from build123d import *

# Parameters (mm, degrees)
SKETCH_1_W          = 30
SKETCH_1_H          = 22
EXTRUDE_1_DEPTH     = 1
SKETCH_2_R          = 0.5
SKETCH_2_R_2        = 0.75
CUT_EXTRUDE_1_DEPTH = 38.215588132
SKETCH_3_W          = 3
SKETCH_3_H          = 10
EXTRUDE_2_DEPTH     = 1
SKETCH_4_R          = 0.5
CUT_EXTRUDE_2_DEPTH = 1


with BuildPart() as part:
    # ｽｹｯﾁ1 → ﾎﾞｽ - 押し出し1 (new body)
    with BuildSketch(Plane.XY):
        with Locations((15, 11)):
            Rectangle(SKETCH_1_W, SKETCH_1_H)
    extrude(amount=EXTRUDE_1_DEPTH)

    # ｽｹｯﾁ2 → ｶｯﾄ - 押し出し1 (cut, through all)
    with BuildSketch(Plane.XY.offset(1)):
        with Locations((4, 17.25)):
            Circle(SKETCH_2_R)
        with Locations((4, 14.71)):
            Circle(SKETCH_2_R)
        with Locations((4, 12.17)):
            Circle(SKETCH_2_R)
        with Locations((4, 9.63)):
            Circle(SKETCH_2_R)
        with Locations((4, 7.09)):
            Circle(SKETCH_2_R)
        with Locations((4, 4.55)):
            Circle(SKETCH_2_R)
        with Locations((26.19, 18.69)):
            Circle(SKETCH_2_R_2)
        with Locations((26.19, 13.61)):
            Circle(SKETCH_2_R_2)
        with Locations((26.19, 8.53)):
            Circle(SKETCH_2_R_2)
        with Locations((26.19, 3.45)):
            Circle(SKETCH_2_R_2)
    extrude(amount=-CUT_EXTRUDE_1_DEPTH, mode=Mode.SUBTRACT)

    # ｽｹｯﾁ3 → ﾎﾞｽ - 押し出し2 (add)
    with BuildSketch(Plane.XY.offset(1)):
        with Locations((15.5, 11)):
            Rectangle(SKETCH_3_W, SKETCH_3_H)
    extrude(amount=EXTRUDE_2_DEPTH)

    # ｽｹｯﾁ4 → ｶｯﾄ - 押し出し2 (cut)
    with BuildSketch(Plane.XY.offset(2)):
        with Locations((15.5, 6)):
            Circle(SKETCH_4_R)
    extrude(amount=-CUT_EXTRUDE_2_DEPTH, mode=Mode.SUBTRACT)


solid = part.part
Design review of the part built by this model. Coordinates are the model's own, in mm. A direction names the side the tool comes from. Coordinates: 2 decimals unless noted, no trailing zeros. Loops run counter-clockwise (first coordinate to the right, second up) from the corner with the lowest first, then second, coordinate; pieces in that order, holes last. Notation, with made-up numbers: M 16.25,-35 L 45.25,-35 A25 ccw 45.25,-14 Z; hole C -6,-3 d5. An arc over 180 degrees is marked long. Use one line per item in the form item = value.
(1) Clearance check with flat-ended pins moving along their axes: P1, Ø0.5, axis at y = 11, z = 1.5, coming from the -X side; P2, Ø1.1, axis at y = 12.5, z = 1.5, coming from the +X side; P3, Ø0.5, axis at x = 16.5, z = 1.5, coming from the -Y side; P4, Ø6.5, axis at x = 21.5, y = 15, coming from the +Z side. State where each tip first meets the part, or that it passes through.
Return value:
P1 = 14
P2 = 30
P3 = 6
P4 = 1
(2) For faces 1 (the face through (17, 10.9, 1.5)), 2 (the face through (15.5, 16, 1.5)), 3 (the face through (15.5, 6.5, 1.5)), 4 (the face through (14, 10.9, 1.5)), list the 3-axis set-ups (+Z, -Z, +X, -X, +Y, -Y) from which the entire face can be reached by the end or side of a thin tool; tool diameter is ignored.
Return value:
face_1 = +Z, +X, +Y, -Y
face_2 = +Z, +X, -X, +Y
face_3 = +Z, -Y
face_4 = +Z, -X, +Y, -Y
(3) Consider section B-B (x = 26.19). Write out the cut boundary in (y, z), and give its area (3 significant figures).
Return value:
outline = M 0,0 L 2.7,0 L 2.7,1 L 0,1 Z; M 4.2,0 L 7.78,0 L 7.78,1 L 4.2,1 Z; M 9.28,0 L 12.86,0 L 12.86,1 L 9.28,1 Z; M 14.36,0 L 17.94,0 L 17.94,1 L 14.36,1 Z; M 19.44,0 L 22,0 L 22,1 L 19.44,1 Z
area = 16.0 mm2
(4) Consider section C-C (z = 0.4). Give the number of separate pieces and of enclosed holes in the cut face, and give its area (3 significant figures).
Return value:
separate_pieces = 1
enclosed_holes = 10
area = 648 mm2
(5) For line 1 along Y through (x, z) = (26.19, 0.35); line 2 along Z through (x, y) = (23, 5.75); line 3 along X through (y, z) = (8, 0.45), list the stretches that pass through material, from the lowest coordinate up. Write a range as from..to.
Return value:
line_1 = 0..2.7, 4.2..7.78, 9.28..12.86, 14.36..17.94, 19.44..22
line_2 = 0..1
line_3 = 0..25.66, 26.72..30
(6) Draft analysis for pull direction Y (two halves, no side actions). For faces 5 (the face through (3.935, 17.746, 0.507)), 6 (the face through (0, 10.8, 0.5)), 7 (the face through (14.5, 6, 1.5)), state which applies: pulls with the +Y half, pulls with the -Y half, needs draft (parallel to the pull), parting line crosses it, or undercut.
Return value:
face_5 = undercut
face_6 = needs draft
face_7 = pulls with the -Y half
(7) Consider section D-D (y = 3.45). Write out the cut boundary in (x, z).
Return value:
outline = M 0,0 L 25.44,0 L 25.44,1 L 0,1 Z; M 26.94,0 L 30,0 L 30,1 L 26.94,1 Z
(8) Consider section A-A (y = 17.25). Write out the cut boundary in (x, z).
Return value:
outline = M 0,0 L 3.5,0 L 3.5,1 L 0,1 Z; M 4.5,0 L 30,0 L 30,1 L 4.5,1 Z
